The listing builds one solid part. Answer for the finished solid, in the listing's coordinates (mm). Face numbers are marked on the shaded views. A direction names the side the tool comes from. Give positions to 0.01 mm unless a question says otherwise; leave off trailing zeros. Write each loop counter-clockwise with the first axis right and the second up, starting at its lowest first coordinate (ties: lowest second). Pieces come first, ordered by that corner, then holes. Notation, with made-up numbers: (74.25, 49) - (105.25, 49) arc R20 ccw to (105.25, 53) - close; hole circle Ø8 at (-34.5, 11.25). An arc over 180 degrees is marked (long way). Answer as CSV lines item,"result". Start each with the question number.
(1) Find section C-C (y = 13). Write down the section's boundary in (x, z), then the cut area to 3 significant figures.
(2) Straight lines are drawn through the part: probe 1 along Y at (x, z) = (-1.75, 2.75); probe 2 along X at (y, z) = (5.25, 6.5); probe 3 along Z at (x, y) = (-12.25, 0.25). For each, find the intervals that lie inside material, in ascending order.
(3) Find section D-D (x = 3). Write down the section's boundary in (y, z), then the cut area to 3 significant figures.
(4) For the marked faces 1, 2 and 3, determine the directions among +Z, -Z, +X, -X, +Y, -Y from which every point of the face is accessible in a straight line to the end or side of a thin tool.
(5) For a pull along X with two mould halves and no side action, classify the marked faces 4, 5, 6 and 7 as pulls with the +X half, pulls with the -X half, needs draft (parallel to the pull), parting line crosses it, or undercut.
(6) Find section B-B (z = 6.25). Write down the section's boundary in (x, y).
(7) Each of these flat-tipped pins is pushed along its axis until it touches: pin 1 Ø3.5 at (x, y) = (6.5, 7) entering from -Z; pin 2 Ø2 at (y, z) = (5, 4.5) entering from -X; pin 3 Ø5 at (x, y) = (0.03, -1.36) entering from -Z; pin 4 Ø2.5 at (x, y) = (5.03, 12.64) entering from +Z. Where does it stop, or does it pass through?
(8) Find section A-A (x = -9.75). Write down the section's boundary in (y, z).
Autodesk Inventor part; units mm, degrees
ref_plane "YZ Plane" through (0, 0, 0) normal (1, 0, 0) x (0, 1, 0)
ref_plane "XZ Plane" through (0, 0, 0) normal (0, 1, 0) x (-1, 0, 0)
ref_plane "XY Plane" through (0, 0, 0) normal (0, 0, 1) x (1, 0, 0)
sketch "Boceto1" plane through (0, 0, 0) normal (0, 0, 1) x (1, 0, 0)
  line L0 (-13.9664, 2.6415) -> (9.0336, 2.6415)
  line L1 (9.0336, 2.6415) -> (9.0336, -5.3585)
  line L2 (9.0336, -5.3585) -> (-13.9664, -5.3585)
  line L3 (-13.9664, -5.3585) -> (-13.9664, 2.6415)
  circle A0 centre (-9.9664, -1.3585) radius 1.5
  circle A1 centre (0.0336, -1.3585) radius 1.5
  point P0 (0, 0)
  dimension "d0" = 3
  dimension "d1" = 3
  dimension "d2" = 23
  dimension "d3" = 8
  dimension "d4" = 10
  dimension "d8" = 4
  dimension "d9" = 4
  dimension "d10" = 4
extrude "Extrusión1" add sketch "Boceto1" along normal blind 4
sketch "Boceto2" plane through (0, 0, 4) normal (0, 0, 1) x (1, 0, 0)
  line L0 (-13.9664, -5.3585) -> (9.0336, -5.3585)
  line L1 (9.0336, -5.3585) -> (2.0336, -5.3585)
  line L2 (2.0336, -5.3585) -> (2.0336, 15.6415)
  line L3 (2.0336, 15.6415) -> (9.0336, 15.6415)
  line L4 (9.0336, 15.6415) -> (9.0336, -5.3585)
  point P0 (0, 0)
  dimension "d11" = 7
  dimension "d12" = 21
extrude "Extrusión2" add sketch "Boceto2" along normal blind 3
sketch "Boceto3" plane through (0, 0, 7) normal (0, 0, 1) x (1, 0, 0)
  circle A0 centre (5.0336, 5.6415) radius 1.5
  circle A1 centre (5.0336, 12.6415) radius 1.5
  line L0 (2.0336, 2.6415) -> (-13.9664, 2.6415)
  line L1 (2.0336, 15.6415) -> (2.0336, -5.3585)
  point P0 (0, 0)
  dimension "d15" = 7
  dimension "d16" = 3
  dimension "d17" = 3
  dimension "d18" = 3
  dimension "d19" = 3
  dimension "d20" = 3
extrude "Extrusión3" cut sketch "Boceto3" against normal up to surface (3 mm away)
equation "\"d1\" = d0"
equation "\"d9\" = 0.5 * d3"
equation "\"d10\" = d9"
equation "\"d18\" = d17"
equation "\"d20\" = d19"
properties part number "Soporte Switch X Izq" material "Acero, fundido"
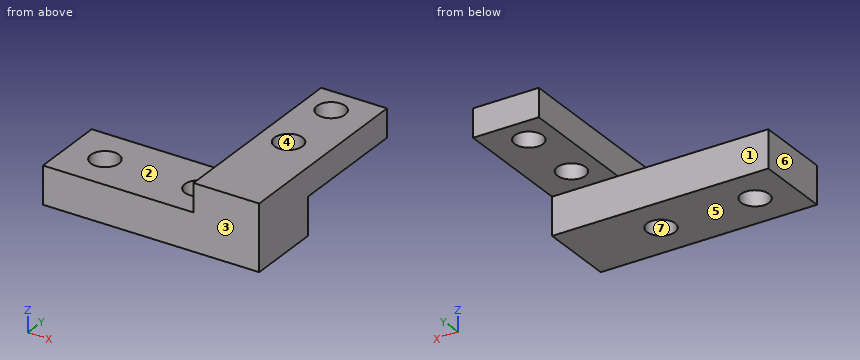
Result set:
1,outline,"(2.03, 4) - (3.58, 4) - (3.58, 7) - (2.03, 7) - close; (6.49, 4) - (9.03, 4) - (9.03, 7) - (6.49, 7) - close"
1,area,"12.3 mm^2"
2,probe 1,"-5.36 to 2.64"
2,probe 2,"2.03 to 3.59, 6.48 to 9.03"
2,probe 3,"0 to 4"
3,outline,"(-5.36, 0) - (2.64, 0) - (2.64, 4) - (15.64, 4) - (15.64, 7) - (-5.36, 7) - close"
3,area,"95.0 mm^2"
4,face 1,"-Z, +X, -X, +Y"
4,face 2,"+Z, -X, +Y, -Y"
4,face 3,"+Z, -Z, +X, -X, -Y"
5,face 4,"undercut"
5,face 5,"needs draft"
5,face 6,"pulls with the -X half"
5,face 7,"undercut"
6,outline,"(2.03, -5.36) - (9.03, -5.36) - (9.03, 15.64) - (2.03, 15.64) - close; hole circle Ø3 at (5.03, 5.64); hole circle Ø3 at (5.03, 12.64)"
7,pin 1,"z = 4"
7,pin 2,"x = 2.03"
7,pin 3,"z = 0"
7,pin 4,"through"
8,outline,"(-5.36, 0) - (-2.84, 0) - (-2.84, 4) - (-5.36, 4) - close; (0.13, 0) - (2.64, 0) - (2.64, 4) - (0.13, 4) - close"
